Answer from the drawing. Dimensions are ordinates in mm from the lowest x, y and z of the part. A direction names the side the tool comes from. Coordinates: 2 decimals unless noted, no trailing zeros. Write each loop counter-clockwise with the first axis right and the second up, starting at its lowest first coordinate (ties: lowest second). Pieces come first, ordered by that corner, then holes. Notation, with made-up numbers: (26.25, 24.25) - (72.25, 24.25) arc R37 ccw to (72.25, 60.25) - close; hole circle Ø1 at (24.25, -35). An arc over 180 degrees is marked (long way). Use a Markdown table: item, result.
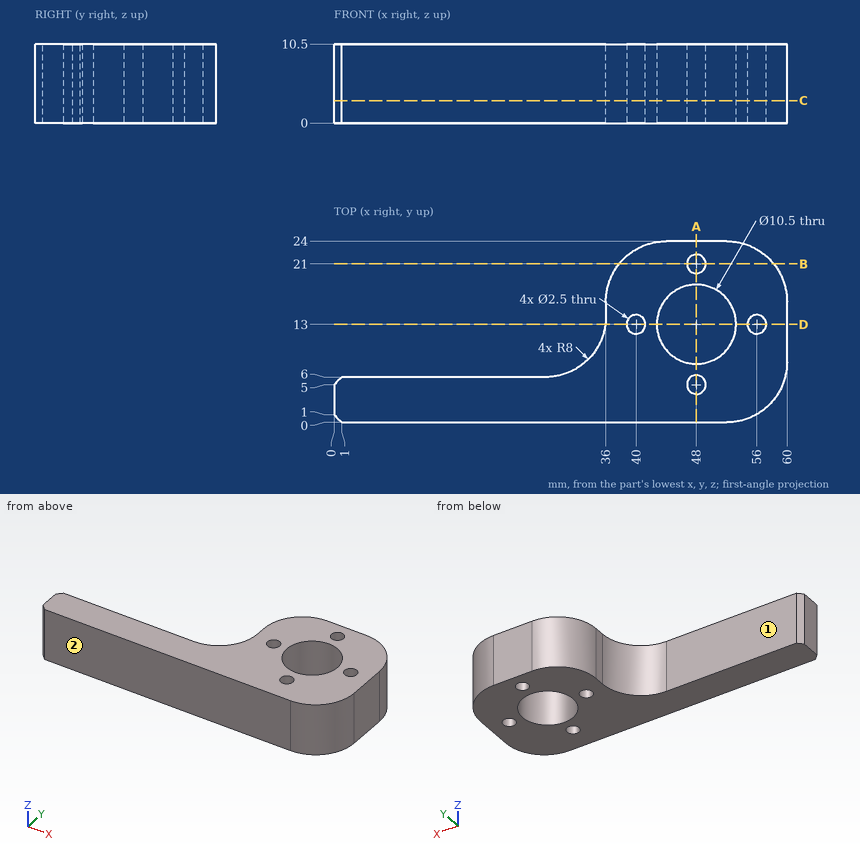
(1) A cutting plane is placed at A-A, the plane x = 48. Write down the section's boundary in (y, z).
Report:
| item | result |
|---|---|
| outline | (0, 0) - (3.75, 0) - (3.75, 10.5) - (0, 10.5) - close; (6.25, 0) - (7.75, 0) - (7.75, 10.5) - (6.25, 10.5) - close; (18.25, 0) - (19.75, 0) - (19.75, 10.5) - (18.25, 10.5) - close; (22.25, 0) - (24, 0) - (24, 10.5) - (22.25, 10.5) - close |
(2) Straight lines are drawn through the part: L1, parallel to Y at x = 48, z = 5.5; L2, parallel to Y at x = 14, z = 7.25; L3, parallel to X at y = 11.5, z = 3.25. For each, find the intervals that lie inside material, in ascending order.
Report:
| item | result |
|---|---|
| L1 | y = 0 to 3.75, 6.25 to 7.75, 18.25 to 19.75, 22.25 to 24 |
| L2 | y = 0 to 6 |
| L3 | x = 35.6 to 42.97, 53.03 to 60 |
(3) Each of these flat-tipped pins is pushed along its axis until it touches: P1, Ø2, axis at x = 23, y = 7.5, coming from the +Z side; P2, Ø1, axis at y = 18.5, z = 7, coming from the -X side; P3, Ø1, axis at y = 15, z = 3, coming from the -X side; P4, Ø2, axis at x = 53.5, z = 2.5, coming from the -Y side. Where does it stop, or does it pass through?
Report:
| item | result |
|---|---|
| P1 | passes through |
| P2 | stops at x = 36.25 |
| P3 | stops at x = 36 |
| P4 | stops at y = 0.02 |
(4) A cutting plane is placed at D-D, the plane y = 13. Write down the section's boundary in (x, z).
Report:
| item | result |
|---|---|
| outline | (35.94, 0) - (38.75, 0) - (38.75, 10.5) - (35.94, 10.5) - close; (41.25, 0) - (42.75, 0) - (42.75, 10.5) - (41.25, 10.5) - close; (53.25, 0) - (54.75, 0) - (54.75, 10.5) - (53.25, 10.5) - close; (57.25, 0) - (60, 0) - (60, 10.5) - (57.25, 10.5) - close |
(5) A cutting plane is placed at B-B, the plane y = 21. Write down the section's boundary in (x, z) (3 decimals).
Report:
| item | result |
|---|---|
| outline | (37.755, 0) - (46.75, 0) - (46.75, 10.5) - (37.755, 10.5) - close; (49.25, 0) - (58.245, 0) - (58.245, 10.5) - (49.25, 10.5) - close |
(6) For the marked faces 1 and 2, determine the directions among +Z, -Z, +X, -X, +Y, -Y from which every point of the face is accessible in a straight line to the end or side of a thin tool.
Report:
| item | result |
|---|---|
| face 1 | +Z, -Z, -X, +Y |
| face 2 | +Z, -Z, +X, -X, -Y |
(7) A cutting plane is placed at C-C, the plane z = 3. Write down the section's boundary in (x, y), and give its area (3 significant figures).
Report:
| item | result |
|---|---|
| outline | (0, 1) - (1, 0) - (52, 0) arc R8 ccw to (60, 8) - (60, 16) arc R8 ccw to (52, 24) - (44, 24) arc R8 ccw to (36, 16) - (36, 14) arc R8 cw to (28, 6) - (1, 6) - (0, 5) - close; hole circle Ø2.5 at (40, 13); hole circle Ø10.5 at (48, 13); hole circle Ø2.5 at (48, 5); hole circle Ø2.5 at (48, 21); hole circle Ø2.5 at (56, 13) |
| area | 657 mm² |
